```python
from build123d import *

# Parameters (mm, degrees)
F0_W     = 95
F0_H     = 5.6
F0_W_2   = 90
F0_H_2   = 2.6
F1_DEPTH = 10
F2_DEPTH = 1.5
F4_DEPTH = 5.6


with BuildPart() as f1:
    # F0 (on Top) → F1 (new body)
    with BuildSketch(Plane.XY):
        Rectangle(F0_W, F0_H)
        Rectangle(F0_W_2, F0_H_2, mode=Mode.SUBTRACT)
    extrude(amount=F1_DEPTH)

    # F0 (on Top) → F2 (join)
    with BuildSketch(Plane.XY):
        Rectangle(F0_W_2, F0_H_2)
    extrude(amount=F2_DEPTH)

    # F3 (on face) → F4 (join)
    with BuildSketch(Plane(origin=(0, 2.8, 0), x_dir=(-1, 0, 0), z_dir=(0, 1, 0))):
        Polygon((-40, -2.3), (-40, 0), (-47.5, 0), (-47.5, -10), (-40, -10), (-40, -7.7), (-45.4, -7.7), (-45.4, -2.3), align=None)
        Polygon((-38, -10), (-38, 0), (-40, 0), (-40, -2.3), (-40, -7.7), (-40, -10), align=None)
        Polygon((40, -2.3), (40, 0), (38, 0), (38, -10), (40, -10), (40, -7.7), align=None)
        Polygon((47.5, 0), (40, 0), (40, -2.3), (45.4, -2.3), (45.4, -7.7), (40, -7.7), (40, -10), (47.5, -10), align=None)
    extrude(amount=-F4_DEPTH)


solid = f1.part
```
Can you work these out from the model? Positions are in its coordinate system, mm. A direction names the side the tool comes from. Give positions to 0.01 mm unless a question says otherwise; leave off trailing zeros. Loops run counter-clockwise (first coordinate to the right, second up) from the corner with the lowest first, then second, coordinate; pieces in that order, holes last. Notation, with made-up numbers: M 7,9 L 50,9 A18 ccw 50,21 Z; hole C -25,81 d5. An arc over 180 degrees is marked long. Use CSV: the item, a comma, the result in double quotes. Start each with the question number.
1. If I drill on L1, parallel to X at y = 0.9, z = -4.75; L2, parallel to X at y = -0.45, z = 9; L3, parallel to Y at x = -1, z = 3.5, over which ranges is the centre line in solid material (lowest first)?
2. Imagine slicing it at C-C, the plane y = 0.3. Write out the boundary of the cut face in (x, z), plus the area to 3 significant figures.
3. Imagine slicing it at A-A, the plane z = -6.75. Write out the boundary of the cut face in (x, y), plus the area to 3 significant figures.
4. Imagine slicing it at D-D, the plane x = -39. Write out the boundary of the cut face in (y, z).
5. Imagine slicing it at B-B, the plane z = 5.5. Write out the boundary of the cut face in (x, y), plus the area to 3 significant figures.
6. For P1, Ø3, axis at x = 5.5, y = 0.5, coming from the -Z side, with a flat end and sliding along its axis, tell me the tip position at first contact or that it passes through.
7. If we mould it in two halves opening along X, with no side actions, what happens to faces 4 (the face through (-47.5, 0, 0)), 5 (the face through (-40, 0, -5)), 6 (the face through (1, 2.8, 5))? For each: released by +X, released by -X, zero draft, split by the parting line, or undercut.
8. On a 3-axis mill with a long thin cutter (end or side, diameter ignored), from which of +Z, -Z, +X, -X, +Y, -Y can I reach the whole of each face in a straight line? I mean faces 1 (the face through (-1, 1.3, 6)), 2 (the face through (43, 0, -2.3)), 3 (the face through (-38, 0, -5)). Say none if no direction works.
Response values:
1,L1,"-47.5 to -45.4, -40 to -38, 38 to 40, 45.4 to 47.5"
1,L2,"-47.5 to -45, 45 to 47.5"
1,L3,"-2.8 to -1.3, 1.3 to 2.8"
2,outline,"M -47.5,-10 L -38,-10 L -38,0 L 38,0 L 38,-10 L 47.5,-10 L 47.5,10 L 45,10 L 45,1.5 L -45,1.5 L -45,10 L -47.5,10 Z; hole M -45.4,-7.7 L -40,-7.7 L -40,-2.3 L -45.4,-2.3 Z; hole M 40,-7.7 L 45.4,-7.7 L 45.4,-2.3 L 40,-2.3 Z"
2,area,"317 mm^2"
3,outline,"M -47.5,-2.8 L -45.4,-2.8 L -45.4,2.8 L -47.5,2.8 Z; M -40,-2.8 L -38,-2.8 L -38,2.8 L -40,2.8 Z; M 38,-2.8 L 40,-2.8 L 40,2.8 L 38,2.8 Z; M 45.4,-2.8 L 47.5,-2.8 L 47.5,2.8 L 45.4,2.8 Z"
3,area,"45.9 mm^2"
4,outline,"M -2.8,-10 L 2.8,-10 L 2.8,10 L 1.3,10 L 1.3,1.5 L -1.3,1.5 L -1.3,10 L -2.8,10 Z"
5,outline,"M -47.5,-2.8 L 47.5,-2.8 L 47.5,2.8 L -47.5,2.8 Z; hole M -45,-1.3 L 45,-1.3 L 45,1.3 L -45,1.3 Z"
5,area,"298 mm^2"
6,P1,"z = 0"
7,face 4,"released by -X"
7,face 5,"undercut"
7,face 6,"zero draft"
8,face 1,"+Z"
8,face 2,"+Y, -Y"
8,face 3,"-Z, +Y, -Y"
